Can you work these out from the model? Positions are in its coordinate system, mm. A direction names the side the tool comes from. Give positions to 0.01 mm unless a question says otherwise; leave off trailing zeros. Loops run counter-clockwise (first coordinate to the right, second up) from the corner with the lowest first, then second, coordinate; pieces in that order, holes last. Notation, with made-up numbers: (67.5, -15.5) - (115.5, -15.5) arc R13 cw to (115.5, 9.5) - close; hole circle Ø4 at (72.25, 28.5). An arc over 180 degrees is marked (long way). Use a Markdown table: item, result. Add a question column.
```python
from build123d import *

# Parameters (mm, degrees)
BASE_FLANGE1_DEPTH = 220
SKETCH6_R          = 1.8
CUT_EXTRUDE1_DEPTH = 343.171009877
SKETCH7_R          = 1.5
CUT_EXTRUDE2_DEPTH = 341.743305143
SKETCH8_R          = 3
CUT_EXTRUDE3_DEPTH = 2
SKETCH10_W         = 100
SKETCH10_H         = 25
CUT_EXTRUDE8_DEPTH = 2
FILLET1_R          = 5
SKETCH11_R         = 5.05
CUT_EXTRUDE9_DEPTH = 2


# Sheet-metal steps are written as plain solids
with BuildPart() as part:
    # Sketch1 → Base-Flange1 (new body)
    with BuildSketch(Plane.XY):
        with BuildLine():
            Line((0, 0), (0, 37))
            ThreePointArc((0, 37), (-0.292893219, 37.707106781), (-1, 38))
            Line((-1, 38), (-25, 38))
            ThreePointArc((-25, 38), (-25.707106781, 37.707106781), (-26, 37))
            Line((-26, 37), (-26, 26))
            ThreePointArc((-26, 26), (-26.878679656, 23.878679656), (-29, 23))
            Line((-29, 23), (-259, 23))
            Line((-259, 23), (-259, 25))
            Line((-259, 25), (-29, 25))
            ThreePointArc((-29, 25), (-28.292893219, 25.292893219), (-28, 26))
            Line((-28, 26), (-28, 37))
            ThreePointArc((-28, 37), (-27.121320344, 39.121320344), (-25, 40))
            Line((-25, 40), (-1, 40))
            ThreePointArc((-1, 40), (1.121320344, 39.121320344), (2, 37))
            Line((2, 37), (2, 0))
            Line((2, 0), (0, 0))
        make_face()
    extrude(amount=BASE_FLANGE1_DEPTH)

    # Sketch6 → Cut-Extrude1 (cut, through all)
    with BuildSketch(Plane(origin=(0, 40, 0), x_dir=(1, 0, 0), z_dir=(0, 1, 0))):
        with Locations(Location((-21, -110, 0), (0, 0, 180))):
            Circle(SKETCH6_R)
        with Locations(Location((-5, -110, 0), (0, 0, 90))):
            Circle(SKETCH6_R)
        with Locations(Location((-13, -118, 0), (0, 0, 180))):
            Circle(SKETCH6_R)
        with Locations(Location((-13, -102, 0), (0, 0, 90))):
            Circle(SKETCH6_R)
    extrude(amount=-CUT_EXTRUDE1_DEPTH, mode=Mode.SUBTRACT)

    # Sketch7 → Cut-Extrude2 (cut, through all)
    with BuildSketch(Plane(origin=(0, 25, 0), x_dir=(1, 0, 0), z_dir=(0, 1, 0))):
        with Locations(Location((-42.5, -5.5, 0), (0, 0, 180))):
            Circle(SKETCH7_R)
        with Locations((-251.5, -5.5)):
            Circle(SKETCH7_R)
        with Locations(Location((-251.5, -214.5, 0), (0, 0, 180))):
            Circle(SKETCH7_R)
        with Locations((-42.5, -214.5)):
            Circle(SKETCH7_R)
    extrude(amount=-CUT_EXTRUDE2_DEPTH, mode=Mode.SUBTRACT)

    # Sketch8 → Cut-Extrude3 (cut)
    with BuildSketch(Plane(origin=(2, 0, 0), x_dir=(0, 0, -1), z_dir=(1, 0, 0))):
        with Locations((-207, 8)):
            Circle(SKETCH8_R)
        with Locations((-207, 29)):
            Circle(SKETCH8_R)
        with Locations(Location((-179, 29, 0), (0, 0, 180))):
            Circle(SKETCH8_R)
        with Locations(Location((-179, 8, 0), (0, 0, 180))):
            Circle(SKETCH8_R)
        with Locations((-41, 8)):
            Circle(SKETCH8_R)
        with Locations((-41, 29)):
            Circle(SKETCH8_R)
        with Locations(Location((-13, 29, 0), (0, 0, 180))):
            Circle(SKETCH8_R)
        with Locations(Location((-13, 8, 0), (0, 0, 180))):
            Circle(SKETCH8_R)
    extrude(amount=-CUT_EXTRUDE3_DEPTH, mode=Mode.SUBTRACT)

    # Sketch10 → Cut-Extrude8 (cut)
    with BuildSketch(Plane(origin=(2, 0, 0), x_dir=(0, 0, -1), z_dir=(1, 0, 0))):
        with Locations((-110, 12.5)):
            Rectangle(SKETCH10_W, SKETCH10_H)
    extrude(amount=-CUT_EXTRUDE8_DEPTH, mode=Mode.SUBTRACT)

    # Fillet1
    fillet1_edges = [part.edges().sort_by_distance(p)[0] for p in [
        (1, 0, 60),
        (1, 0, 160),
        (1, 25, 160),
        (1, 25, 60),
    ]]
    fillet(fillet1_edges, radius=FILLET1_R)

    # Sketch11 → Cut-Extrude9 (cut)
    with BuildSketch(Plane(origin=(0, 40, 0), x_dir=(1, 0, 0), z_dir=(0, 1, 0))):
        with Locations(Location((-13, -110, 0), (0, 0, 270))):
            Circle(SKETCH11_R)
    extrude(amount=-CUT_EXTRUDE9_DEPTH, mode=Mode.SUBTRACT)


solid = part.part
```
1. Suppose I cut it at A-A (y = 29). List the corners of the cut face in (x, z) for me, and give its area (3 significant figures).
2. If we mould it in two halves opening along Z, with no side actions, what happens to faces 1 (the face through (1, 8, 210)), 2 (the face through (-12.778, 39.014, 104.955)), 3 (the face through (-142, 23, 108)), 4 (the face through (-137.6, 24.5, 0))? For each: released by +Z, released by -Z, zero draft, split by the parting line, or undercut.
3. Suppose I cut it at B-B (z = 207). List the corners of the cut face in (x, y) for me.
4. On a 3-axis mill with a long thin cutter (end or side, diameter ignored), from which of +Z, -Z, +X, -X, +Y, -Y can I reach the whole of each face in a straight line? I mean faces 5 (the face through (0, 26, 108)), 6 (the face through (1, 8, 44)), 7 (the face through (-146, 25, 108)), 8 (the face through (1, 29, 210)). Say none if no direction works.
5. Will these pins go through, and if not, where does the flat tip stop? P1, Ø4, axis at x = -42.5, z = 5.5, coming from the -Y side; P2, Ø5, axis at y = 8, z = 41, coming from the -X side; P3, Ø5, axis at x = -78.5, z = 126, coming from the +Y side; P4, Ø4.5, axis at x = -13, z = 102, coming from the -Y side.
6. Please list where these lines run through material, in increasing order: line 1 along Z through (x, y) = (-42.5, 24.45); line 2 along X through (y, z) = (26, 154); line 3 along X through (y, z) = (39, 110). Write a range as [from, to].
7. Suppose I cut it at D-D (x = -242). List the corners of the cut face in (y, z) for me, and give its area (3 significant figures).
8. Suppose I cut it at C-C (y = 8). List the corners of the cut face in (x, z) for me, and give its area (3 significant figures).
Results below:
| question | item | result |
|---|---|---|
| 1 | outline | (-28, 0) - (-26, 0) - (-26, 220) - (-28, 220) - close; (0, 0) - (2, 0) - (2, 10) - (0, 10) - close; (0, 16) - (2, 16) - (2, 38) - (0, 38) - close; (0, 44) - (2, 44) - (2, 176) - (0, 176) - close; (0, 182) - (2, 182) - (2, 204) - (0, 204) - close; (0, 210) - (2, 210) - (2, 220) - (0, 220) - close |
| 1 | area | 832 mm² |
| 2 | face 1 | undercut |
| 2 | face 2 | undercut |
| 2 | face 3 | zero draft |
| 2 | face 4 | released by -Z |
| 3 | outline | (-259, 23) - (-29, 23) arc R3 ccw to (-26, 26) - (-26, 37) arc R1 cw to (-25, 38) - (-1, 38) arc R1 cw to (0, 37) - (0, 32) - (2, 32) - (2, 37) arc R3 ccw to (-1, 40) - (-25, 40) arc R3 ccw to (-28, 37) - (-28, 26) arc R1 cw to (-29, 25) - (-259, 25) - close; (0, 0) - (2, 0) - (2, 5) - (0, 5) - close; (0, 11) - (2, 11) - (2, 26) - (0, 26) - close |
| 4 | face 5 | +Z, -Z, -Y |
| 4 | face 6 | +X, -X |
| 4 | face 7 | +Z, -Z, -X, +Y |
| 4 | face 8 | +X |
| 5 | P1 | y = 23 |
| 5 | P2 | through |
| 5 | P3 | y = 25 |
| 5 | P4 | y = 38 |
| 6 | line 1 | [0, 4], [7, 213], [216, 220] |
| 6 | line 2 | [-28, -26], [0, 2] |
| 6 | line 3 | [-27.24, -22.8], [-19.2, -18.05], [-7.95, -6.8], [-3.2, 1.24] |
| 7 | outline | (23, 0) - (25, 0) - (25, 220) - (23, 220) - close |
| 7 | area | 440 mm² |
| 8 | outline | (0, 0) - (2, 0) - (2, 10) - (0, 10) - close; (0, 16) - (2, 16) - (2, 38) - (0, 38) - close; (0, 44) - (2, 44) - (2, 60) - (0, 60) - close; (0, 160) - (2, 160) - (2, 176) - (0, 176) - close; (0, 182) - (2, 182) - (2, 204) - (0, 204) - close; (0, 210) - (2, 210) - (2, 220) - (0, 220) - close |
| 8 | area | 192 mm² |
